from build123d import *

# Parameters (mm, degrees)
SKETCH_1_R      = 2.75
SKETCH_1_R_2    = 4
EXTRUDE_1_DEPTH = 5
SKETCH_2_R      = 10
SKETCH_2_R_2    = 4.15
EXTRUDE_2_DEPTH = 5
FILLET_1_R      = 5


with BuildPart() as part:
    # 草图1 → 凸台-拉伸1 (new body)
    with BuildSketch(Plane(origin=(0, 0, 0), x_dir=(1, 0, 0), z_dir=(0, 1, 0))):
        with BuildLine():
            Line((10, 0), (10, 33.5))
            Line((10, 33.5), (-10, 33.5))
            Line((-10, 33.5), (-10, 0))
            ThreePointArc((-10, 0), (0, -10), (10, 0))
        make_face()
        with Locations(Location((0, 27.5, 0), (0, 0, 270))):
            Circle(SKETCH_1_R, mode=Mode.SUBTRACT)
        with Locations(Location((0, 15.5, 0), (0, 0, 270))):
            Circle(SKETCH_1_R, mode=Mode.SUBTRACT)
        with Locations(Location((0, 0, 0), (0, 0, 270))):
            Circle(SKETCH_1_R_2, mode=Mode.SUBTRACT)
    extrude(amount=EXTRUDE_1_DEPTH)

    # 草图2 → 凸台-拉伸2 (add)
    with BuildSketch(Plane(origin=(0, 5, 0), x_dir=(1, 0, 0), z_dir=(0, 1, 0))):
        Circle(SKETCH_2_R)
        with Locations(Location((0, 0, 0), (0, 0, 270))):
            Circle(SKETCH_2_R_2, mode=Mode.SUBTRACT)
    extrude(amount=EXTRUDE_2_DEPTH)

    # 圆角1
    fillet_1_edges = [part.edges().sort_by_distance(p)[0] for p in [
        (-10, 2.5, -33.5),
        (10, 2.5, -33.5),
    ]]
    fillet(fillet_1_edges, radius=FILLET_1_R)


solid = part.part
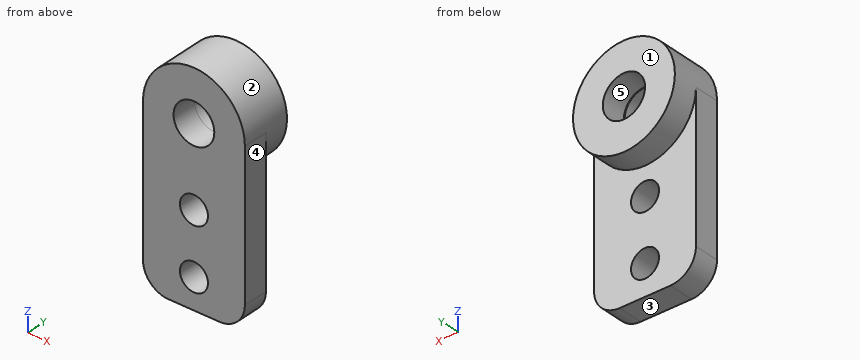
Input: part model. Units: mm. Frame: model coordinates. Face numbers are marked on the shaded views. A direction names the side the tool comes from. Round coordinates to 2 decimals unless told otherwise and drop trailing zeros. Order: outer loops, then holes, each group sorted by start corner. A loop starts at its lowest first (then second) coordinate and runs counter-clockwise, first axis right, second up. Notation, with made-up numbers: (-20, 25) - (16, 25) arc R21 ccw to (16, 55) - close; hole circle Ø10 at (22.5, 30.5). An arc over 180 degrees is marked (long way). Answer as a JSON object with one key per item and string values. Group by question number.
(1) Material intervals for probe 1 along X at (y, z) = (8.7, 0); probe 2 along X at (y, z) = (4.75, -27.5); probe 3 along Y at (x, z) = (-8.25, -11), sorted ascending. Write a range as from..to.
(2) Reachability of the marked faces 1 and 2 from +Z, -Z, +X, -X, +Y, -Y: full face, straight path, thin tool, end or side. Return the list, or none.
(3) Pin query (flat end, axial travel): P1, Ø1, axis at x = -5, y = 4, coming from the +Z side; P2, Ø6.5, axis at x = 2, z = 0, coming from the +Y side; P3, Ø4, axis at x = 6, z = -10.5, coming from the +Y side. Return the tip coordinate at first contact, or that it passes through.
(4) Cut plane B-B (y = 1). Return loops of the section in (x, z), then the cut area to 3 significant figures.
(5) Cut plane D-D (y = 5.5). Return loops of the section in (x, z).
(6) Cut plane C-C (x = -1.5). Return loops of the section in (y, z), then the cut area to 3 significant figures.
(7) Cut plane A-A (z = -27.5). Return loops of the section in (x, y), then the cut area to 3 significant figures.
(8) Draft query along Z for the marked faces 3, 4 and 5. Return one class per face: released by +Z, released by -Z, zero draft, split by the parting line, or undercut.
Here are the results:
{
 "1": {"probe 1": "x = -10..-4.15, 4.15..10", "probe 2": "x = -10..-2.75, 2.75..10", "probe 3": "y = 0..5"},
 "2": {"face 1": "+Z, -Z, +X, -X, +Y", "face 2": "+Y"},
 "3": {"P1": "stops at z = 8.93", "P2": "stops at y = 10", "P3": "stops at y = 5"},
 "4": {"outline": "(-10, -28.5) arc R5 ccw to (-5, -33.5) - (5, -33.5) arc R5 ccw to (10, -28.5) - (10, 0) arc R10 ccw to (-10, 0) - close; hole circle Ø8 at (0, 0); hole circle Ø5.5 at (0, -27.5); hole circle Ø5.5 at (0, -15.5)", "area": "719 mm^2"},
 "5": {"outline": "circle Ø20 at (0, 0); hole circle Ø8.3 at (0, 0)"},
 "6": {"outline": "(0, -33.5) - (5, -33.5) - (5, -29.8) - (0, -29.8) - close; (0, -25.2) - (5, -25.2) - (5, -17.8) - (0, -17.8) - close; (0, -13.2) - (5, -13.2) - (5, -9.89) - (10, -9.89) - (10, -3.87) - (5, -3.87) - (5, -3.71) - (0, -3.71) - close; (0, 3.71) - (5, 3.71) - (5, 3.87) - (10, 3.87) - (10, 9.89) - (0, 9.89) - close", "area": "194 mm^2"},
 "7": {"outline": "(-10, 0) - (-2.75, 0) - (-2.75, 5) - (-10, 5) - close; (2.75, 0) - (10, 0) - (10, 5) - (2.75, 5) - close", "area": "72.5 mm^2"},
 "8": {"face 3": "released by -Z", "face 4": "zero draft", "face 5": "undercut"}
}
